Source: three-view drawing plus pictorial views. Frame: mm from the lowest corner of the part. Give positions to 0.01 mm unless a question says otherwise; leave off trailing zeros. Write each loop counter-clockwise with the first axis right and the second up, starting at its lowest first coordinate (ties: lowest second). Pieces come first, ordered by that corner, then holes.
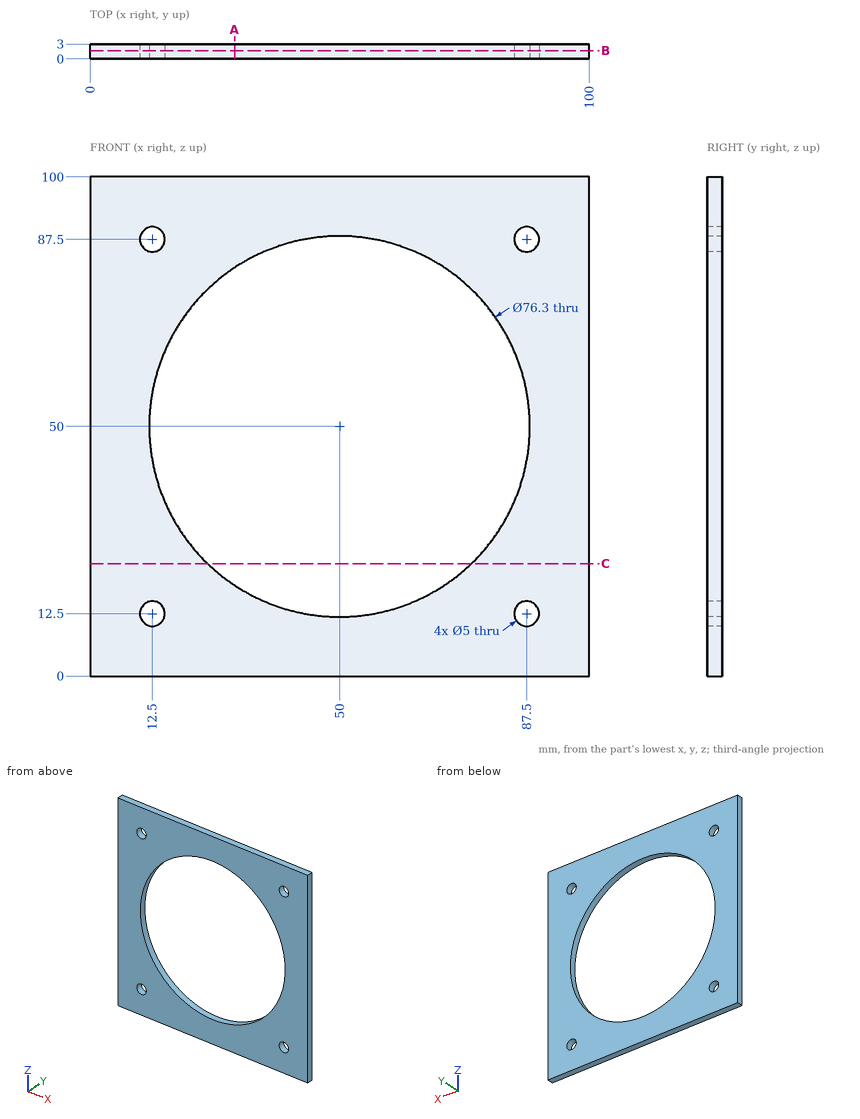
Q1. Section C-C on z = 22.5. Output: boundary loops of the cut face in (x, y), plus the area to 3 significant figures.
Filled sheet:
outline: (0, 0) - (23.56, 0) - (23.56, 3) - (0, 3) - close; (76.44, 0) - (100, 0) - (100, 3) - (76.44, 3) - close
area: 141 mm2
Q2. Pin query (flat end, axial travel): P1, Ø3, axis at x = 12.5, z = 12.5, coming from the -Y side. Return the tip coordinate at first contact, or that it passes through.
Filled sheet:
P1: passes through
Q3. Section A-A on x = 29. Output: boundary loops of the cut face in (y, z), plus the area to 3 significant figures.
Filled sheet:
outline: (0, 0) - (3, 0) - (3, 18.15) - (0, 18.15) - close; (0, 81.85) - (3, 81.85) - (3, 100) - (0, 100) - close
area: 109 mm2
Q4. Ray query, line 1 along Z through (x, y) = (50, 2.05); line 2 along Z through (x, y) = (63, 0.45); line 3 along X through (y, z) = (2, 44). Return the intervals inside material, ascending.
Filled sheet:
line 1: z = 0 to 11.85, 88.15 to 100
line 2: z = 0 to 14.13, 85.87 to 100
line 3: x = 0 to 12.32, 87.68 to 100
Q5. Section B-B on y = 1.65. Output: boundary loops of the cut face in (x, z), plus the area to 3 significant figures.
Filled sheet:
outline: (0, 0) - (100, 0) - (100, 100) - (0, 100) - close; hole circle Ø5 at (12.5, 12.5); hole circle Ø5 at (12.5, 87.5); hole circle Ø76.3 at (50, 50); hole circle Ø5 at (87.5, 12.5); hole circle Ø5 at (87.5, 87.5)
area: 5,350 mm2
